Geometry: final body of the model. Coordinates: model frame, mm. Face numbers are marked on the shaded views. A direction names the side the tool comes from. Coordinates: 2 decimals unless noted, no trailing zeros. Write each loop counter-clockwise with the first axis right and the second up, starting at its lowest first coordinate (ties: lowest second). Pieces come first, ordered by that corner, then holes. Notation, with made-up numbers: M 52,-35 L 80,-35 A19 cw 80,-1 Z; hole C 15.5,70 d6. An arc over 180 degrees is marked long. Write item = value, one per line. Start each with the question number.
Item 1: Section C-C on y = -11.5. Output: boundary loops of the cut face in (x, z).
Item 2: Section B-B on z = 2.5. Output: boundary loops of the cut face in (x, y).
Item 3: Ray query, L1, parallel to Z at x = 0, y = 5.65; L2, parallel to X at y = 5.6, z = 0; L3, parallel to Z at x = 0, y = 5.3. Return the intervals inside material, ascending. Write a range as [from, to].
Item 4: Section D-D on x = -6.5. Output: boundary loops of the cut face in (y, z), plus the area to 3 significant figures.
Item 5: Reachability of the marked faces 1, 2, 3 and 4 from +Z, -Z, +X, -X, +Y, -Y: full face, straight path, thin tool, end or side. Return the list, or none.
Item 6: First-contact query: pin 1 Ø6 at (y, z) = (-4.5, -3.5) entering from +X; pin 2 Ø4.5 at (x, z) = (-1.5, 1) entering from +Y; pin 3 Ø4 at (x, y) = (1.5, -18) entering from +Z. Flat tips, straight axial feed; report the tip coordinate or a pass-through.
Item 7: Pull-direction query (X, two-part tool) for the marked faces 5, 6, 7 and 8; classes: +X half, -X half, draft (parallel to the pull), parting line (faces both ways), or undercut.
Item 8: Section A-A on x = 0. Output: boundary loops of the cut face in (y, z).
Autodesk Inventor part; units mm, degrees
ref_plane "YZ Plane" through (0, 0, 0) normal (1, 0, 0) x (0, 1, 0)
ref_plane "XZ Plane" through (0, 0, 0) normal (0, 1, 0) x (-1, 0, 0)
ref_plane "XY Plane" through (0, 0, 0) normal (0, 0, 1) x (1, 0, 0)
sketch "Boceto1" plane through (0, 0, 0) normal (0, 1, 0) x (-1, 0, 0)
  circle A0 centre (0, 0) radius 7.5
  dimension "d0" = 15
extrude "Extrusión1" add sketch "Boceto1" along normal blind 1
sketch "Boceto2" plane through (0, 1, 0) normal (0, 1, 0) x (1, 0, 0)
  line L0 (-3.4641, 6) -> (3.4641, 6)
  line L1 (3.4641, 6) -> (6.9282, 0)
  line L2 (6.9282, 0) -> (3.4641, -6)
  line L3 (3.4641, -6) -> (-3.4641, -6)
  line L4 (-3.4641, -6) -> (-6.9282, 0)
  line L5 (-6.9282, 0) -> (-3.4641, 6)
  point P0 (0, 0)
  point P1 (0, 0)
  dimension "d3" = 6
  dimension "d4" = 0
extrude "Extrusión2" add sketch "Boceto2" along normal blind 5
sketch "Boceto3" plane through (0, 0, 0) normal (0, -1, 0) x (1, 0, 0)
  circle A0 centre (0, 0) radius 5
  dimension "d7" = 10
extrude "Extrusión3" add sketch "Boceto3" along normal blind 21
sketch "Boceto5" plane through (0, -21, 0) normal (0, -1, 0) x (1, 0, 0)
  circle A0 centre (0, 0) radius 3.5
  dimension "d15" = 7
extrude "Extrusión4" add sketch "Boceto5" along normal blind 11
thread "Rosca2"
chamfer "Chaflán1" distance 1 angle 45 6 edges at (-5.1962, 6, -3) (0, 6, -6) (5.1962, 6, -3) (5.1962, 6, 3) (0, 6, 6) (-5.1962, 6, 3)
sketch "Boceto6" plane through (0, 6, 0) normal (0, 1, 0) x (1, 0, 0)
  circle A0 centre (0, 0) radius 4.5
  dimension "d23" = 9
extrude "Extrusión5" cut sketch "Boceto6" against normal blind 1
properties part number "BASE_PERNO"
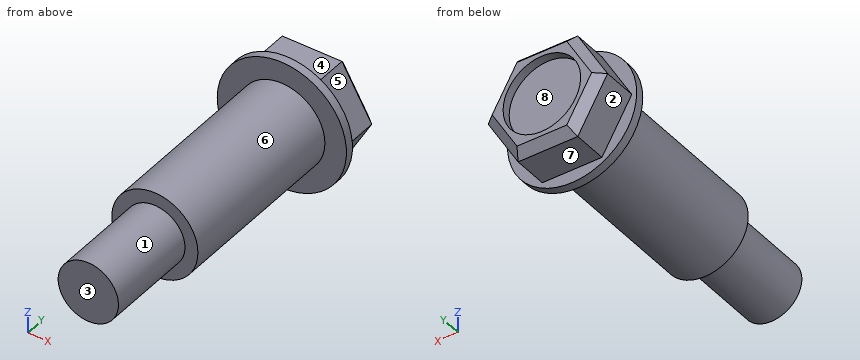
Responses:
q1.outline = C 0,0 d10
q2.outline = M -7.07,0 L -4.33,0 L -4.33,-21 L -2.45,-21 L -2.45,-32 L 2.45,-32 L 2.45,-21 L 4.33,-21 L 4.33,0 L 7.07,0 L 7.07,1 L 5.48,1 L 5.48,5 L 4.33,6 L 3.74,6 L 3.74,5 L -3.74,5 L -3.74,6 L -4.33,6 L -5.48,5 L -5.48,1 L -7.07,1 Z
q3.L1 = [-5.35, -4.5], [4.5, 5.35]
q3.L2 = [-6.24, -4.5], [4.5, 6.24]
q3.L3 = [-5.7, -4.5], [4.5, 5.7]
q4.outline = M 0,-3.74 L 1,-3.74 L 1,-0.74 L 5,-0.74 L 5.37,0 L 5,0.74 L 1,0.74 L 1,3.74 L 0,3.74 Z
q4.area = 13.7 mm²
q5.face_1 = -Y
q5.face_2 = -Z, -X, +Y
q5.face_3 = +Z, -Z, +X, -X, -Y
q5.face_4 = +Z, +X, -X, +Y
q6.pin_1 = 4.97
q6.pin_2 = 5
q6.pin_3 = 5
q7.face_5 = +X half
q7.face_6 = parting line
q7.face_7 = draft
q7.face_8 = undercut
q8.outline = M -32,-3.5 L -21,-3.5 L -21,-5 L 0,-5 L 0,-7.5 L 1,-7.5 L 1,-6 L 5,-6 L 6,-5 L 6,-4.5 L 5,-4.5 L 5,4.5 L 6,4.5 L 6,5 L 5,6 L 1,6 L 1,7.5 L 0,7.5 L 0,5 L -21,5 L -21,3.5 L -32,3.5 Z
